Part model, mm, in its own coordinate system. Round coordinates to 2 decimals unless told otherwise and drop trailing zeros. Loops run counter-clockwise (first coordinate to the right, second up) from the corner with the lowest first, then second, coordinate; pieces in that order, holes last.
from build123d import *

# Parameters (mm, degrees)
ESQUISSE1_R             = 27.5
BOSS_EXTRU_1_DEPTH      = 20
ESQUISSE2_R             = 27.5
BOSS_EXTRU_2_DEPTH      = 50
ESQUISSE3_R             = 16.05
ENL_V_MAT_EXTRU_1_DEPTH = 51


with BuildPart() as part:
    # Esquisse1 → Boss.-Extru.1 (new body)
    with BuildSketch(Plane.XY):
        Circle(ESQUISSE1_R)
    extrude(amount=BOSS_EXTRU_1_DEPTH)

    # Esquisse2 → Boss.-Extru.2 (add)
    with BuildSketch(Plane.XY):
        Circle(ESQUISSE2_R)
    extrude(amount=BOSS_EXTRU_2_DEPTH)

    # Esquisse3 → Enlèv. mat.-Extru.1 (cut, through all)
    with BuildSketch(Plane(origin=(0, 0, 0), x_dir=(-1, 0, 0), z_dir=(0, 0, -1))):
        Circle(ESQUISSE3_R)
    extrude(amount=-ENL_V_MAT_EXTRU_1_DEPTH, mode=Mode.SUBTRACT)


solid = part.part
1) Mould opens along X. For faces 1 (the face through (12.737, -9.766, 24.65)), 2 (the face through (-5.961, -26.846, 24.65)), 3 (the face through (12, -12, 50)) say: released by +X, released by -X, zero draft, split by the parting line, or undercut.
Values:
face 1: undercut
face 2: split by the parting line
face 3: zero draft
2) Slice it at A-A, the plane x = 0. Give the cut face in (y, z), then the cut area to 4 significant figures.
Values:
outline: (-27.5, 0) - (-16.05, 0) - (-16.05, 50) - (-27.5, 50) - close; (16.05, 0) - (27.5, 0) - (27.5, 50) - (16.05, 50) - close
area: 1,145 mm2
3) Wall check: line 1 along Y through (x, z) = (0, 28.5); line 2 along X through (y, z) = (-8.5, 46); line 3 along X through (y, z) = (2.5, 37). Give the ranges that are in metal, low to high.
Values:
line 1: y = -27.5 to -16.05, 16.05 to 27.5
line 2: x = -26.15 to -13.61, 13.61 to 26.15
line 3: x = -27.39 to -15.85, 15.85 to 27.39
4) Drop flat-ended pins along their axis: pin 1 Ø1.5 at (x, z) = (7, 16) entering from +Y; pin 2 Ø2 at (y, z) = (10.5, 38.5) entering from -X; pin 3 Ø2 at (y, z) = (9.5, 27) entering from +X. Give the stop position or say it passes through.
Values:
pin 1: stops at y = 26.78
pin 2: stops at x = -25.81
pin 3: stops at x = 26.15
5) Slice it at D-D, the plane y = 17.5. Give the cut face in (x, z), then the cut area to 3 significant figures.
Values:
outline: (-21.21, 0) - (21.21, 0) - (21.21, 50) - (-21.21, 50) - close
area: 2,120 mm2
6) Slice it at C-C, the plane z = 18.5. Give the cut face in (x, y), then the cut area to 3 significant figures.
Values:
outline: circle Ø55 at (0, 0); hole circle Ø32.1 at (0, 0)
area: 1,570 mm2
